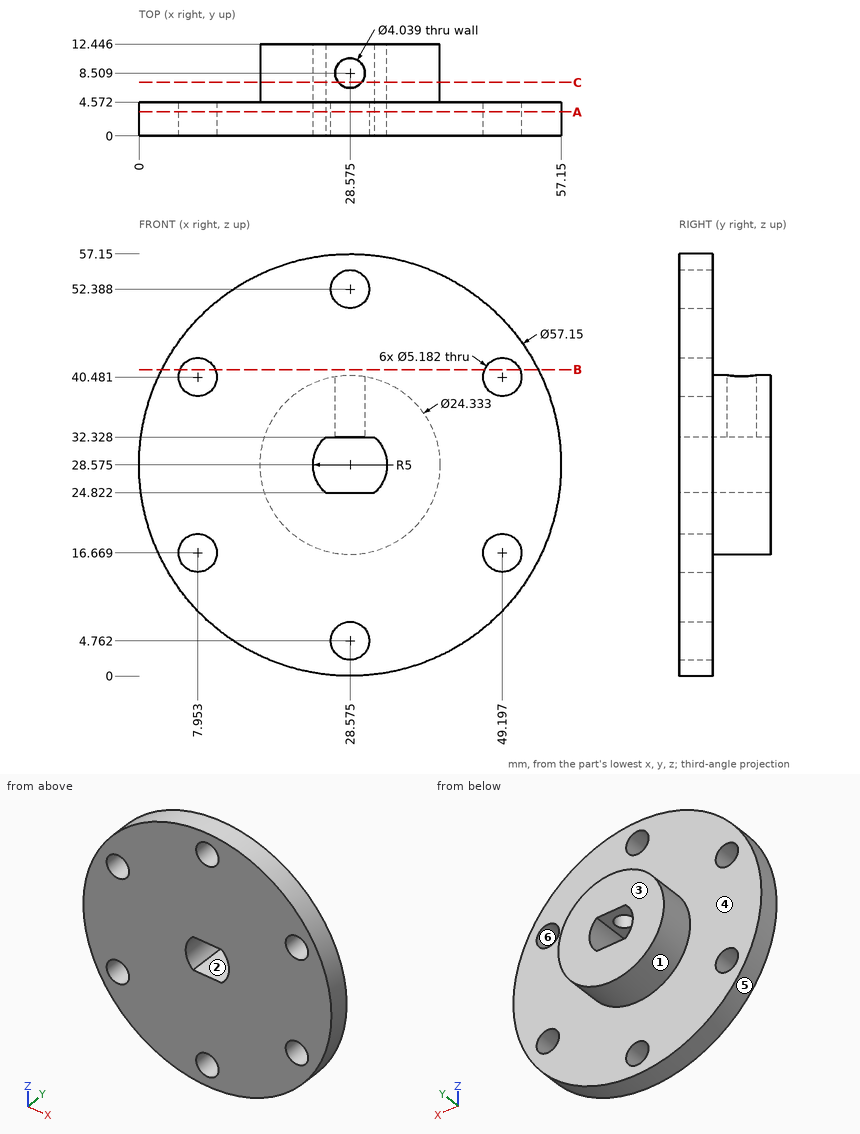
The figure shows three views and two pictorial views of one solid part (mm, origin at its lowest corner). Answer the questions. A direction names the side the tool comes from. Give positions to 0.01 mm unless a question says otherwise; leave off trailing zeros. Write each loop counter-clockwise with the first axis right and the second up, starting at its lowest first coordinate (ties: lowest second). Pieces come first, ordered by that corner, then holes. Notation, with made-up numbers: M -26.5,-37.5 L 23.5,-37.5 A28 cw 23.5,-15.5 Z; hole C 26,-32 d9. An arc over 180 degrees is marked long. Write each question's results on one line, items separated by ' | '.
Q1. For a pull along Z with two mould halves and no side action, classify the marked faces 4, 5 and 6 as released by +Z, released by -Z, zero draft, split by the parting line, or undercut.
Output values:
face 4: zero draft | face 5: split by the parting line | face 6: undercut
Q2. Section A-A, the plane y = 3.25 is taken. Count the separate pieces of the cut face and the enclosed holes in it, then the cut area to 3 significant figures.
Output values:
separate pieces: 1 | enclosed holes: 7 | area: 2,370 mm2
Q3. Section B-B, the plane z = 41.5 is taken. Write down the section's boundary in (x, y) (1 decimal).
Output values:
outline: M 3.1,0 L 5.6,0 L 5.6,4.6 L 3.1,4.6 Z; M 10.3,0 L 46.8,0 L 46.8,4.6 L 10.3,4.6 Z; M 51.6,0 L 54.1,0 L 54.1,4.6 L 51.6,4.6 Z
Q4. A tool of negligible diameter and unlimited length cuts with its end or side. For the marked faces 1, 2 and 3, from which of +Z, -Z, +X, -X, +Y, -Y can it reach the whole face along a straight path? Write none if from no direction.
Output values:
face 1: +Y | face 2: +Y, -Y | face 3: +Z, -Z, +X, -X, +Y
Q5. Consider L1, parallel to Z at x = 7.5, y = 2 (1 decimal); L2, parallel to Y at x = 42, z = 5; L3, parallel to Z at x = 6, y = 3.25 (1 decimal). Determine where each line is inside the solid, lowest interval first. Write a range as from..to.
Output values:
L1: 9.3..14.1, 19.2..37.9, 43..47.9 | L2: 0..4.57 | L3: 11.1..15, 18.4..38.8, 42.2..46.1
Q6. Section C-C, the plane y = 7.25 is taken. Write down the section's boundary in (x, z) (1 decimal).
Output values:
outline: M 25.3,24.8 A5 cw 25.3,32.3 L 27,32.3 L 27,40.6 A12.2 ccw long 30.2,40.6 L 30.2,32.3 L 31.9,32.3 A5 cw 31.9,24.8 Z
Q7. Flat-ended cylindrical pins translate along their axes: P1, Ø4, axis at x = 41, z = 51, coming from the +Y side; P2, Ø1, axis at y = 5, z = 26, coming from the -X side; P3, Ø2.5, axis at x = 28.575, y = 8.509, coming from the -Z side; P4, Ø12, axis at x = 51.5, z = 30, coming from the -Y side. Find the tip coordinate at first contact, or state that the pin passes through.
Output values:
P1: y = 4.57 | P2: x = 0.09 | P3: z = 16.41 | P4: y = 0
